Can you work these out from the drawing? Everything is in mm from the part's minimum corner. A direction names the side the tool comes from. Round coordinates to 2 decimals unless told otherwise and drop trailing zeros. Order: outer loops, then holes, each group sorted by start corner. A loop starts at its lowest first (then second) coordinate and runs counter-clockwise, first axis right, second up. Notation, with made-up numbers: (70, 63) -> (87, 63) arc R26 ccw to (87, 77) -> close; hole circle Ø10 at (28.25, -27.5). An arc over 180 degrees is marked (long way). One line per item, written item: value.
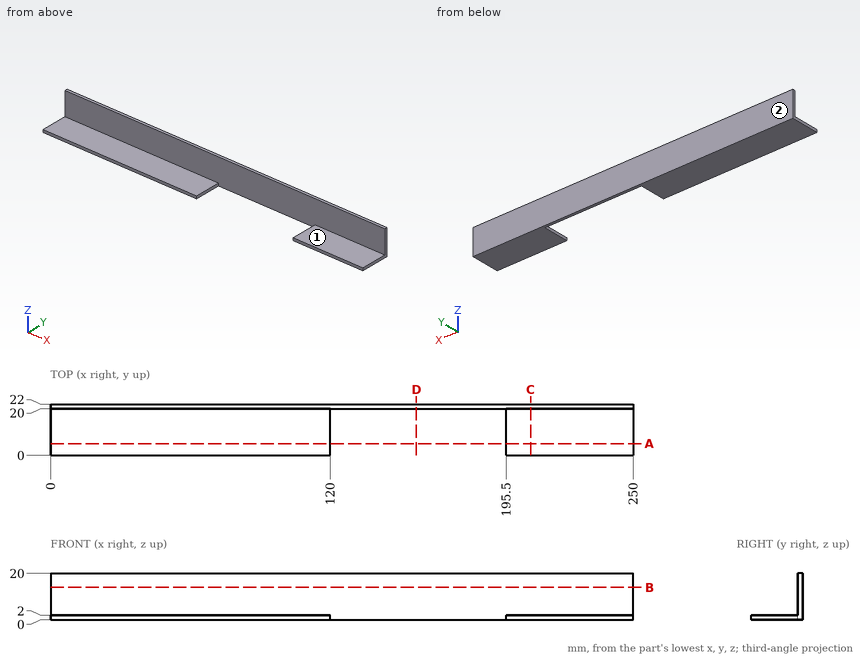
Q1. I want a section at B-B on z = 14. Write out the boundary of the cut face in (x, y).
Answers:
outline: (0, 20) -> (250, 20) -> (250, 22) -> (0, 22) -> close
Q2. Which directions (+Z, -Z, +X, -X, +Y, -Y) give clear straight access to the entire face, cutting with the end or side of a thin tool? Please do the marked faces 1 and 2.
Answers:
face 1: +Z, +X, -X, -Y
face 2: +Z, -Z, +X, -X, +Y
Q3. For P1, Ø10, axis at x = 152.5, z = 10.5, coming from the -Y side; P2, Ø3, axis at y = 17.5, z = 17, coming from the -X side; P3, Ø10, axis at x = 44, y = 11, coming from the +Z side, each with a flat end and sliding along its axis, tell me the tip position at first contact or that it passes through.
Answers:
P1: y = 20
P2: through
P3: z = 2
Q4. I need wall thicknesses on line 1 along X through (y, z) = (14.25, 1); line 2 along Z through (x, y) = (210, 16.75); line 3 along Y through (x, z) = (71.5, 10.25). Which ranges of each line are inside material? Lowest first, please.
Answers:
line 1: 0 to 120, 195.5 to 250
line 2: 0 to 2
line 3: 20 to 22
Q5. I want a section at C-C on x = 206. Write out the boundary of the cut face in (y, z), then the cut area to 3 significant figures.
Answers:
outline: (0, 0) -> (22, 0) -> (22, 20) -> (20, 20) -> (20, 2) -> (0, 2) -> close
area: 80.0 mm2
Q6. I want a section at A-A on y = 5. Write out the boundary of the cut face in (x, z), then the cut area to 3 significant figures.
Answers:
outline: (0, 0) -> (120, 0) -> (120, 2) -> (0, 2) -> close; (195.5, 0) -> (250, 0) -> (250, 2) -> (195.5, 2) -> close
area: 349 mm2
Q7. I want a section at D-D on x = 157. Write out the boundary of the cut face in (y, z).
Answers:
outline: (20, 0) -> (22, 0) -> (22, 20) -> (20, 20) -> close
